Job drawing, mm, ordinate dimensions from the low corner. One solid piece. A direction names the side the tool comes from. Coordinates: 2 decimals unless noted, no trailing zeros. Order: outer loops, then holes, each group sorted by start corner. A loop starts at its lowest first (then second) coordinate and runs counter-clockwise, first axis right, second up. Notation, with made-up numbers: (76.25, 76.25) - (111.25, 76.25) arc R10 ccw to (111.25, 91.25) - close; hole circle Ø6 at (19, -17). An arc over 180 degrees is marked (long way). Use one line per item in the form item = value.
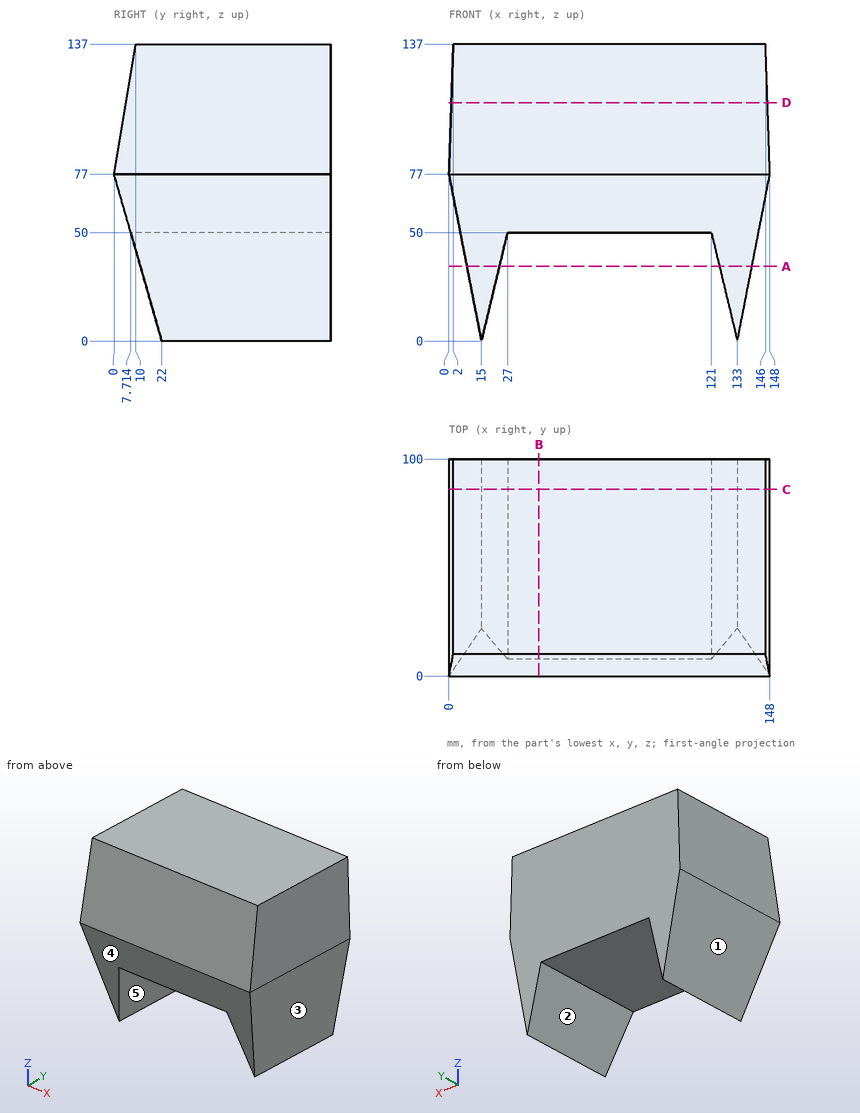
Item 1: Drop flat-ended pins along their axis: pin 1 (1 mm diameter, centred on y = 26.5, z = 70.5, fed in from -X); pin 2 (1.5 mm diameter, centred on x = 45.5, y = 36.5, fed in from -Z); pin 3 (10 mm diameter, centred on y = 50, z = 71, fed in from -X) (1 decimal). Give the stop position or say it passes through.
Derived:
pin_1 = 1.17
pin_2 = 50
pin_3 = 0.2
Item 2: Cut at B-B, the plane x = 41.5. Write the cut outline in (y, z), plus the area to 3 significant figures.
Derived:
outline = (0, 77) - (7.71, 50) - (100, 50) - (100, 137) - (10, 137) - close
area = 8,300 mm²
Item 3: Drill centre lines: line 1 (Z direction, x = 51, y = 87); line 2 (X direction, y = 55, z = 44); line 3 (X direction, y = 55, z = 35). Where is each one in solid material? Low to high. Write a range as [from, to].
Derived:
line_1 = [50, 137]
line_2 = [6.43, 25.56], [122.44, 141.57]
line_3 = [8.18, 23.4], [124.6, 139.82]
Item 4: Cut at A-A, the plane z = 34.5. Write the cut outline in (x, y), plus the area to 3 significant figures.
Derived:
outline = (8.28, 12.14) - (23.28, 12.14) - (23.28, 100) - (8.28, 100) - close; (124.72, 12.14) - (139.72, 12.14) - (139.72, 100) - (124.72, 100) - close
area = 2,640 mm²
Item 5: Cut at C-C, the plane y = 86. Write the cut outline in (x, z).
Derived:
outline = (0, 77) - (15, 0) - (27, 50) - (121, 50) - (133, 0) - (148, 77) - (146, 137) - (2, 137) - close
Item 6: 3-axis set-ups, long thin cutter, end or side, ignore diameter. For the marked faces 4 and 5: which of +Z, -Z, +X, -X, +Y, -Y reach the whole face in a straight line?
Derived:
face_4 = -Z, +X, -X, -Y
face_5 = -Z, +Y, -Y
Item 7: Cut at D-D, the plane z = 110. Write the cut outline in (x, y).
Derived:
outline = (1.1, 5.5) - (146.9, 5.5) - (146.9, 100) - (1.1, 100) - close
Item 8: Two-plate mould, pull along X, no slides. Class the marked faces 1, 2 and 3: +X half, -X half, draft (parallel to the pull), parting line (faces both ways), or undercut.
Derived:
face_1 = -X half
face_2 = undercut
face_3 = +X half
